Design review of the part built by this model. Coordinates are the model's own, in mm. A direction names the side the tool comes from. Round coordinates to 2 decimals unless told otherwise and drop trailing zeros. Loops run counter-clockwise (first coordinate to the right, second up) from the corner with the lowest first, then second, coordinate; pieces in that order, holes last. Notation, with made-up numbers: (10.25, 61) - (24.25, 61) arc R23 cw to (24.25, 98) - close; hole circle Ø10 at (26.25, 15). An arc over 180 degrees is marked (long way). Use one line per item in the form item = value. Start each with the question number.
(1) For pin 1 (9 mm diameter, centred on x = -127, z = 31.75, fed in from +Y); pin 2 (3 mm diameter, centred on x = 98.5, y = 4, fed in from -Z); pin 3 (5 mm diameter, centred on x = -57.63, z = -195.03, fed in from -Y); pin 4 (1.5 mm diameter, centred on x = -30, y = 4.5, fed in from +Z), all flat-tipped, find the tip position at first contact; note any pin that passes through.
(2) The part is to be moulded in two halves that separate along Z. For faces 3 (the flat face through (-4, 6.35, 53)), 4 (the flat face through (-84, 0, 7.144)), 5 (the cylindrical face through (-55.06, 0.09, 247.96)), say which applies: released by +Z, released by -Z, zero draft, split by the parting line, or undercut.
(3) We need section B-B, the plane y = 0.25. Give the number of separate pieces and of enclosed holes in the cut face, then the cut area to 3 significant figures.
(4) Machinability: for faces 1 (the flat face through (-4, -3.175, 11)), 2 (the flat face through (71.801, 0.089, 43.336)), which of the approach directions +Z, -Z, +X, -X, +Y, -Y give a long, thin tool a straight path to every point of the face, cutting with its end or side? Answer none if there is none.
(5) We need section C-C, the plane z = -173. Write out the cut boundary in (x, y), then the cut area to 3 significant figures.
(6) Wall thickness on probe 1 along Z at (x, y) = (-55, 5); probe 2 along X at (y, z) = (4, 20); probe 3 along Z at (x, y) = (56.5, 5.25): over which ranges is each line inside the solid? List them lowest first. Write a range as [from, to].
(7) We need section A-A, the plane x = -190. Write out the cut boundary in (y, z), then the cut area to 3 significant figures.
from build123d import *

# Parameters (mm, degrees)
SKETCH1_R                                = 254
BOSS_EXTRUDE1_DEPTH                      = 6.35
F_10_CLEARANCE_HOLE1_D                   = 5.6134
F_10_CLEARANCE_HOLE1_DEPTH               = 12.7
SKETCH3_W                                = 39.6875
SKETCH3_H                                = 14.2875
SKETCH3_W_2                              = 26.9875
CUT_EXTRUDE2_DEPTH                       = 13.7
F_1_4_CLEARANCE_HOLE1_D                  = 6.7564
F_1_4_0_2500_DOWEL_HOLE2_D               = 6.35
CIRPATTERN1_COUNT                        = 5
CBORE_FOR_1_4_HEX_HEAD_BOLT1_D           = 22.86
CBORE_FOR_1_4_HEX_HEAD_BOLT1_CBORE_D     = 31.75
CBORE_FOR_1_4_HEX_HEAD_BOLT1_CBORE_DEPTH = 3.175


with BuildPart() as part:
    # Sketch1 → Boss-Extrude1 (new body, symmetric)
    with BuildSketch(Plane(origin=(0, 0, 0), x_dir=(1, 0, 0), z_dir=(0, 1, 0))):
        Circle(SKETCH1_R)
    extrude(amount=BOSS_EXTRUDE1_DEPTH, both=True)

    # #10 Clearance Hole1
    with Locations(Plane(origin=(0, 6.35, 0), x_dir=(1, 0, 0), z_dir=(0, 1, 0))):
        with Locations((-11.90625, 20.622229928), (11.90625, 20.622229928), (23.8125, 0), (11.90625, -20.622229928), (-11.90625, -20.622229928), (-23.8125, 0)):
            Hole(F_10_CLEARANCE_HOLE1_D / 2, depth=F_10_CLEARANCE_HOLE1_DEPTH)

    # Sketch3 → Cut-Extrude2 (cut, through all)
    with BuildSketch(Plane(origin=(0, 6.35, 0), x_dir=(1, 0, 0), z_dir=(0, 1, 0))):
        with Locations((-83.34375, 0)):
            Rectangle(SKETCH3_W, SKETCH3_H)
        with Locations((-215.10625, 0)):
            Rectangle(SKETCH3_W_2, SKETCH3_H)
    cut_extrude2 = extrude(amount=-CUT_EXTRUDE2_DEPTH, mode=Mode.SUBTRACT)

    # 1/4 Clearance Hole1 (through all)
    with Locations(Plane(origin=(0, 6.35, 0), x_dir=(1, 0, 0), z_dir=(0, 1, 0))):
        with Locations((-158.75, -31.75), (-127, -31.75)):
            f_1_4_clearance_hole1 = Hole(F_1_4_CLEARANCE_HOLE1_D / 2)

    # 1/4 (0.2500) Dowel Hole2 (through all)
    with Locations(Plane(origin=(0, 6.35, 0), x_dir=(1, 0, 0), z_dir=(0, 1, 0))):
        with Locations((-65.183798023, 5.459951977), (-65.183798023, -5.459951977), (-101.503701977, -5.459951977), (-101.503701977, 5.459951977), (-203.296298023, 5.459951977), (-203.296298023, -5.459951977), (-226.916201977, -5.459951977), (-226.916201977, 5.459951977)):
            f_1_4_0_2500_dowel_hole2 = Hole(F_1_4_0_2500_DOWEL_HOLE2_D / 2)

    # CirPattern1: Cut-Extrude2, 1/4 Clearance Hole1, 1/4 (0.2500) Dowel Hole2 ×5 about axis
    cirpattern1_axis = Axis((0, 0, 0), (0, 1, 0))
    for i in range(1, CIRPATTERN1_COUNT):
        add(cut_extrude2.rotate(cirpattern1_axis, i * 360 / CIRPATTERN1_COUNT), mode=Mode.SUBTRACT)
        add(f_1_4_clearance_hole1.rotate(cirpattern1_axis, i * 360 / CIRPATTERN1_COUNT), mode=Mode.SUBTRACT)
        add(f_1_4_0_2500_dowel_hole2.rotate(cirpattern1_axis, i * 360 / CIRPATTERN1_COUNT), mode=Mode.SUBTRACT)

    # CBORE for 1/4 Hex Head Bolt1 (through all)
    with Locations(Plane.XZ.offset(6.35)):
        with Locations((0, 0)):
            CounterBoreHole(CBORE_FOR_1_4_HEX_HEAD_BOLT1_D / 2, CBORE_FOR_1_4_HEX_HEAD_BOLT1_CBORE_D / 2, CBORE_FOR_1_4_HEX_HEAD_BOLT1_CBORE_DEPTH)


solid = part.part
Data:
q1.pin_1 = 6.35
q1.pin_2 = -234.75
q1.pin_3 = through
q1.pin_4 = 252.31
q2.face_3 = zero draft
q2.face_4 = undercut
q2.face_5 = split by the parting line
q3.separate_pieces = 1
q3.enclosed_holes = 27
q3.area = 197,000 mm^2
q4.face_1 = -Y
q4.face_2 = +Y, -Y
q5.outline = (-185.98, -6.35) - (185.98, -6.35) - (185.98, 6.35) - (-185.98, 6.35) - close
q5.area = 4,720 mm^2
q6.probe_1 = [-247.97, -196.81], [-193.25, 193.25], [196.81, 247.97]
q6.probe_2 = [-253.21, -14.64], [-9.17, 9.17], [14.64, 253.21]
q6.probe_3 = [-247.64, -49.88], [-30.77, 30.77], [49.88, 247.64]
q7.outline = (-6.35, -168.57) - (6.35, -168.57) - (6.35, 168.57) - (-6.35, 168.57) - close
q7.area = 4,280 mm^2
